Study the drawing (mm; zero at the part's minimum x, y, z) and answer. Give positions to 0.01 mm unless a question says otherwise; leave off trailing zeros. Write each loop counter-clockwise with the first axis right and the second up, starting at its lowest first coordinate (ties: lowest second). Pieces come first, ordered by that corner, then holes. Notation, with made-up numbers: (-21.5, -19.5) - (27.5, -19.5) arc R20 ccw to (27.5, 11.5) - close; hole circle Ø7 at (-11.5, 56). An arc over 180 degrees is marked (long way). Answer in a Markdown table with one row per item. Add a question column.
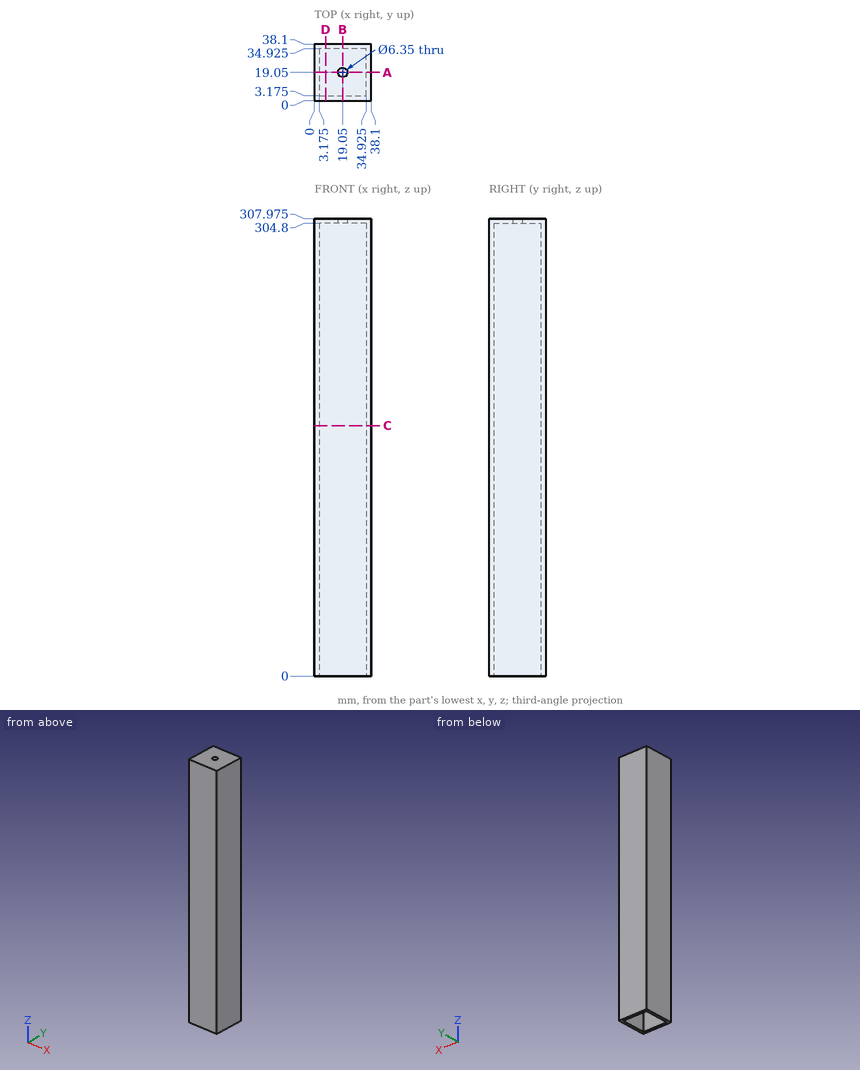
1. Section D-D (x = 7.5) is taken. Give the vertices of the cut face in (y, z) (3 decimals), and give its area (3 significant figures).
2. Section C-C (z = 168.5) is taken. Give the vertices of the cut face in (x, y) (3 decimals), and give its area (3 significant figures).
3. Straight lines are drawn through the part: L1, parallel to X at y = 31, z = 110.5 (3 decimals); L2, parallel to X at y = 19, z = 305. For each, find the intervals that lie inside material, in ascending order. Write a range as [from, to].
4. Given pin 1 Ø9.5 at (x, y) = (15, 22.5) entering from -Z, flat-ended and moving along its own axis, determine where the tip first touches the part or whether it passes through.
5. Section A-A (y = 19.05) is taken. Give the vertices of the cut face in (x, z) (3 decimals), and give its area (3 significant figures).
Geometry check:
| question | item | result |
|---|---|---|
| 1 | outline | (0, 0) - (3.175, 0) - (3.175, 304.8) - (34.925, 304.8) - (34.925, 0) - (38.1, 0) - (38.1, 307.975) - (0, 307.975) - close |
| 1 | area | 2,060 mm² |
| 2 | outline | (0, 0) - (38.1, 0) - (38.1, 38.1) - (0, 38.1) - close; hole (3.175, 3.175) - (34.925, 3.175) - (34.925, 34.925) - (3.175, 34.925) - close |
| 2 | area | 444 mm² |
| 3 | L1 | [0, 3.175], [34.925, 38.1] |
| 3 | L2 | [0, 15.88], [22.22, 38.1] |
| 4 | pin 1 | z = 304.8 |
| 5 | outline | (0, 0) - (3.175, 0) - (3.175, 304.8) - (15.875, 304.8) - (15.875, 307.975) - (0, 307.975) - close; (22.225, 304.8) - (34.925, 304.8) - (34.925, 0) - (38.1, 0) - (38.1, 307.975) - (22.225, 307.975) - close |
| 5 | area | 2,040 mm² |
